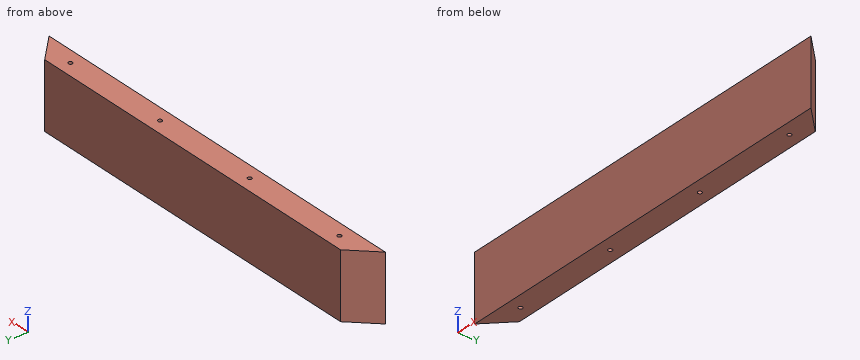
from build123d import *

# Parameters (mm, degrees)
SALIENTE_EXTRUIR1_DEPTH = 250
CROQUIS2_R              = 1.25
CORTAR_EXTRUIR1_DEPTH   = 41


with BuildPart() as part:
    # Croquis1 → Saliente-Extruir1 (new body)
    with BuildSketch(Plane(origin=(0, 0, 0), x_dir=(0, 0, -1), z_dir=(1, 0, 0))):
        Polygon((-20, 0), (20, 0), (20, 15), (18.5, 15), (-18.5, 15), (-20, 15), align=None)
    extrude(amount=SALIENTE_EXTRUIR1_DEPTH)

    # Croquis2 → Cortar-Extruir1 (cut, through all)
    with BuildSketch(Plane(origin=(0, 0, -20), x_dir=(-1, 0, 0), z_dir=(0, 0, -1))):
        with Locations((-225, 7.5)):
            Circle(CROQUIS2_R)
        with Locations((-25, 7.5)):
            Circle(CROQUIS2_R)
        with Locations((-158.333333333, 7.5)):
            Circle(CROQUIS2_R)
        with Locations((-91.666666667, 7.5)):
            Circle(CROQUIS2_R)
        Polygon((0, 15), (-15, 15), (0, 0), align=None)
        Polygon((-250, 15), (-235, 15), (-250, 0), align=None)
    extrude(amount=-CORTAR_EXTRUIR1_DEPTH, mode=Mode.SUBTRACT)


solid = part.part
Verification items for the finished model (mm, model axes). Give positions to 0.01 mm unless a question says otherwise; leave off trailing zeros. Loops run counter-clockwise (first coordinate to the right, second up) from the corner with the lowest first, then second, coordinate; pieces in that order, holes last.
1) Sectioned sample at B-B, the plane y = 11.75. Enter the section's corners in (x, z).
2) Thickness scan on line 1 along Y through (x, z) = (225, -10); line 2 along X through (y, z) = (7, 18.5); line 3 along X through (y, z) = (3.5, 3.5). Record the ranges inside material, lowest first.
3) Sectioned sample at A-A, the plane z = 2.5. Enter the section's corners in (x, y), then the cut area to 3 significant figures.
4) Depth check by flat-ended pin: pin 1 Ø1.5 at (x, y) = (25, 7.5) entering from -Z. Enter the tip coordinate at first touch or a pass-through.
Answers:
1. outline: (11.75, -20) - (238.25, -20) - (238.25, 20) - (11.75, 20) - close
2. line 1: y = 0 to 6.25, 8.75 to 15
2. line 2: x = 7 to 23.85, 26.15 to 90.52, 92.81 to 157.19, 159.48 to 223.85, 226.15 to 243
2. line 3: x = 3.5 to 246.5
3. outline: (0, 0) - (250, 0) - (235, 15) - (15, 15) - close; hole circle Ø2.5 at (25, 7.5); hole circle Ø2.5 at (91.67, 7.5); hole circle Ø2.5 at (158.33, 7.5); hole circle Ø2.5 at (225, 7.5)
3. area: 3,510 mm2
4. pin 1: passes through
